Here's how the part is built. I have some questions about the finished solid (model axes, mm). A direction names the side the tool comes from. Round coordinates to 2 decimals unless told otherwise and drop trailing zeros. Write each loop counter-clockwise with the first axis right and the second up, starting at its lowest first coordinate (ties: lowest second). Pieces come first, ordered by that corner, then holes. Notation, with made-up numbers: M 21,13.5 L 41,13.5 A17 ccw 41,39.5 Z; hole C 7.25,-34 d9. An arc over 180 degrees is marked long. Use a Markdown table: item, result. Add a question column.
```python
from build123d import *

# Parameters (mm, degrees)
BOSS_EXTRUDE1_DEPTH = 162
SKETCH2_R           = 15
CUT_EXTRUDE1_DEPTH  = 15
SKETCH4_W           = 280
SKETCH4_H           = 152
CUT_EXTRUDE3_DEPTH  = 135
FILLET2_R           = 10
FILLET3_R           = 5
SKETCH5_R           = 5
CUT_EXTRUDE4_DEPTH  = 135


with BuildPart() as part:
    # Sketch1 → Boss-Extrude1 (new body)
    with BuildSketch(Plane.XY):
        Polygon((-46.03724142, 83.913559712), (66.03724142, 83.913559712), (160, -66.086440288), (10, -66.086440288), (-140, -66.086440288), align=None)
    extrude(amount=BOSS_EXTRUDE1_DEPTH)

    # Sketch2 → Cut-Extrude1 (cut)
    with BuildSketch(Plane(origin=(0, 83.913559712, 0), x_dir=(1, 0, 0), z_dir=(0, 1, 0))):
        with Locations(Location((10, -81, 0), (0, 0, 180))):
            Circle(SKETCH2_R)
    extrude(amount=-CUT_EXTRUDE1_DEPTH, mode=Mode.SUBTRACT)

    # Sketch4 → Cut-Extrude3 (cut)
    with BuildSketch(Plane.XZ.offset(66.086440288)):
        with Locations((10, 81)):
            Rectangle(SKETCH4_W, SKETCH4_H)
    extrude(amount=-CUT_EXTRUDE3_DEPTH, mode=Mode.SUBTRACT)

    # Fillet2
    fillet2_edges = [part.edges().sort_by_distance(p)[0] for p in [
        (-46.03724142, 83.913559712, 81),
        (66.03724142, 83.913559712, 81),
    ]]
    fillet(fillet2_edges, radius=FILLET2_R)

    # Fillet3
    fillet3_edges = [part.edges().sort_by_distance(p)[0] for p in [
        (160, -66.086440288, 81),
        (-140, -66.086440288, 81),
    ]]
    fillet(fillet3_edges, radius=FILLET3_R)

    # Sketch5 → Cut-Extrude4 (cut)
    with BuildSketch(Plane.XY.offset(162)):
        with Locations((102.275314, -54.350620288)):
            Circle(SKETCH5_R)
        with Locations((-82.275314, -54.350620288)):
            Circle(SKETCH5_R)
    extrude(amount=-CUT_EXTRUDE4_DEPTH, mode=Mode.SUBTRACT)


solid = part.part
```
Item 1: On a 3-axis mill with a long thin cutter (end or side, diameter ignored), from which of +Z, -Z, +X, -X, +Y, -Y can I reach the whole of each face in a straight line? I mean faces 1 (the face through (150, -58, 80)), 2 (the face through (8, -15, 5)), 3 (the face through (-130.62, -51.11, 74.62)), 4 (the face through (-5.5, 68.914, 82.1)), 5 (the face through (-85.96, -50.97, 159.54)). Say none if no direction works.
Item 2: For pin 1 Ø8 at (y, z) = (-57, 58.5) entering from +X, with a flat end and sliding along its axis, tell me the tip position at first contact or that it passes through.
Item 3: I need wall thicknesses on probe 1 along Z at (x, y) = (-102, -42.5); probe 2 along Z at (x, y) = (10, 74); probe 3 along X at (y, z) = (69, 91). Which ranges of each line are inside material? Lowest first, please. Write a range as from..to.
Item 4: Imagine slicing it at D-D on y = 53. List the corners of the cut face in (x, z) for me, plus the area to 3 significant figures.
Item 5: Imagine slicing it at C-C on z = 99. List the corners of the cut face in (x, y) for me, plus the area to 3 significant figures.
Item 6: If we mould it in two halves opening along Z, with no side actions, what happens to faces 6 (the face through (12, -7, 162)), 7 (the face through (13.252, 76.519, 66.357)), 8 (the face through (8, -15, 157)), 9 (the face through (-135.4, -63.4, 82.1))? For each: +Z half, -Z half, draft (parallel to the pull), parting line (faces both ways), or undercut.
Item 7: Imagine slicing it at B-B on x = 10. List the corners of the cut face in (y, z) for me, plus the area to 3 significant figures.
Item 8: Imagine slicing it at A-A on z = 81. List the corners of the cut face in (x, y) for me, plus the area to 3 significant figures.
The answers:
| question | item | result |
|---|---|---|
| 1 | face 1 | +Y, -Y |
| 1 | face 2 | -Y |
| 1 | face 3 | +Z, -Z, -X, +Y |
| 1 | face 4 | +X, -X, -Y |
| 1 | face 5 | +Z |
| 2 | pin 1 | x = 155.97 |
| 3 | probe 1 | 0..5, 157..162 |
| 3 | probe 2 | 0..66, 96..162 |
| 3 | probe 3 | -55.38..-1.18, 21.18..75.38 |
| 4 | outline | M -65.4,0 L 85.4,0 L 85.4,5 L -65.4,5 Z; M -65.4,157 L 85.4,157 L 85.4,162 L -65.4,162 Z |
| 4 | area | 1,510 mm² |
| 5 | outline | M -135.21,-58.43 A5 ccw -130.97,-66.09 L -130,-66.09 L -130,-50.12 Z; M -55.43,68.91 L 75.43,68.91 L 68.98,79.22 A10 ccw 60.5,83.91 L -40.5,83.91 A10 ccw -48.98,79.22 Z; M 150,-66.09 L 150.97,-66.09 A5 ccw 155.21,-58.43 L 150,-50.12 Z |
| 5 | area | 1,940 mm² |
| 6 | face 6 | +Z half |
| 6 | face 7 | undercut |
| 6 | face 8 | undercut |
| 6 | face 9 | draft |
| 7 | outline | M -66.09,0 L 83.91,0 L 83.91,66 L 68.91,66 L 68.91,5 L -66.09,5 Z; M -66.09,157 L 68.91,157 L 68.91,96 L 83.91,96 L 83.91,162 L -66.09,162 Z |
| 7 | area | 3,330 mm² |
| 8 | outline | M -135.21,-58.43 A5 ccw -130.97,-66.09 L -130,-66.09 L -130,-50.12 Z; M -55.43,68.91 L -5,68.91 L -5,83.91 L -40.5,83.91 A10 ccw -48.98,79.22 Z; M 25,68.91 L 75.43,68.91 L 68.98,79.22 A10 ccw 60.5,83.91 L 25,83.91 Z; M 150,-66.09 L 150.97,-66.09 A5 ccw 155.21,-58.43 L 150,-50.12 Z |
| 8 | area | 1,490 mm² |
